from build123d import *

# Parameters (mm, degrees)
SKETCH_R              = 1.6
PAD_DEPTH             = 3
POLARPATTERN_COUNT    = 3
POCKET_DEPTH          = 380.288671
POLARPATTERN001_COUNT = 3
CHAMFER_SIZE          = 1
FILLET_R              = 3
SKETCH066_R           = 1.6
POCKET032_DEPTH       = 3.001
SKETCH078_R           = 3
POCKET038_DEPTH       = 5
POLARPATTERN007_COUNT = 3
CHAMFER017_SIZE       = 3


with BuildPart() as part:
    # Sketch → Pad (new body)
    with BuildSketch(Plane.XY):
        Polygon((0, 0), (-49.917704, 28.82), (-56.37248, 17.64), (-49.641016, 5.980762), (-58.30127, 0.980762), (-71.291651, -6.519238), (-41.291651, -58.480762), (-28.30127, -50.980762), (-19.641016, -45.980762), (-12.909552, -57.64), (0, -57.64), align=None)
        with Locations((-51.471143, -0.849365)):
            Circle(SKETCH_R, mode=Mode.SUBTRACT)
    pad = extrude(amount=PAD_DEPTH)

    # PolarPattern: Pad ×3 about axis
    polarpattern_axis = Axis((0, 0, 0), (0, 0, 1))
    for i in range(1, POLARPATTERN_COUNT):
        add(pad.rotate(polarpattern_axis, i * 360 / POLARPATTERN_COUNT))

    # Sketch001 → Pocket (cut, through all)
    with BuildSketch(Plane.XY):
        Polygon((-28.267069, 16.32), (-37.267069, 0.731543), (-18, -32.64), (0, -32.64), (0, 0), align=None)
    pocket = extrude(amount=POCKET_DEPTH, mode=Mode.SUBTRACT)

    # PolarPattern001: Pocket ×3 about axis
    polarpattern001_axis = Axis((0, 0, 0), (0, 0, 1))
    for i in range(1, POLARPATTERN001_COUNT):
        add(pocket.rotate(polarpattern001_axis, i * 360 / POLARPATTERN001_COUNT), mode=Mode.SUBTRACT)

    # Chamfer
    chamfer_edges = [part.edges().sort_by_distance(p)[0] for p in [
        (-56.37248, 17.64, 1.5),
        (-43.462928, 40, 1.5),
        (43.462928, 40, 1.5),
        (56.37248, 17.64, 1.5),
        (12.909552, -57.64, 1.5),
        (-12.909552, -57.64, 1.5),
    ]]
    chamfer(chamfer_edges, length=CHAMFER_SIZE)

    # Fillet
    fillet_edges = [part.edges().sort_by_distance(p)[0] for p in [
        (-19.267069, 31.908457, 1.5),
        (18, -32.64, 1.5),
        (-18, -32.64, 1.5),
        (37.267069, 0.731543, 1.5),
        (19.267069, 31.908457, 1.5),
        (-37.267069, 0.731543, 1.5),
    ]]
    fillet(fillet_edges, radius=FILLET_R)

    # Sketch066 (on Binder) → Pocket032 (cut, through all)
    with BuildSketch(Plane(origin=(0, 0, 3), x_dir=(1, 0, 0), z_dir=(0, 0, -1))):
        with Locations((-24.348373, 30.5)):
            Circle(SKETCH066_R)
        with Locations((38.587961, 5.836309)):
            Circle(SKETCH066_R)
        with Locations((-14.239588, -36.336309)):
            Circle(SKETCH066_R)
    extrude(amount=POCKET032_DEPTH, mode=Mode.SUBTRACT)

    # Sketch078 (on Face44 of Pocket032) → Pocket038 (cut)
    with BuildSketch(Plane.XY.offset(3)):
        with Locations((25, 45)):
            Circle(SKETCH078_R)
    pocket038 = extrude(amount=-POCKET038_DEPTH, mode=Mode.SUBTRACT)

    # PolarPattern007: Pocket038 ×3 about axis
    polarpattern007_axis = Axis((0, 0, 3), (0, 0, 1))
    for i in range(1, POLARPATTERN007_COUNT):
        add(pocket038.rotate(polarpattern007_axis, i * 360 / POLARPATTERN007_COUNT), mode=Mode.SUBTRACT)

    # Chamfer017
    chamfer017_edges = [part.edges().sort_by_distance(p)[0] for p in [
        (-41.291651, -58.480762, 1.5),
        (-71.291651, -6.519238, 1.5),
        (-30, 65, 1.5),
        (41.291651, -58.480762, 1.5),
        (71.291651, -6.519238, 1.5),
        (30, 65, 1.5),
        (-19.641016, -45.980762, 1.5),
        (49.641016, 5.980762, 1.5),
        (-30, 40, 1.5),
        (30, 40, 1.5),
        (-49.641016, 5.980762, 1.5),
        (19.641016, -45.980762, 1.5),
    ]]
    chamfer(chamfer017_edges, length=CHAMFER017_SIZE)


solid = part.part
Here's how the part is built. I have some questions about the finished solid (model axes, mm). A direction names the side the tool comes from. Round coordinates to 2 decimals unless told otherwise and drop trailing zeros. Write each loop counter-clockwise with the first axis right and the second up, starting at its lowest first coordinate (ties: lowest second). Pieces come first, ordered by that corner, then holes. Notation, with made-up numbers: (62.5, -5.5) -> (73.5, -5.5) arc R19 cw to (73.5, 26.5) -> close; hole circle Ø10 at (68.5, 60.5). An arc over 180 degrees is marked (long way). One line per item, written item: value.
1) We'd pull the mould along Y, two halves only. Please class faces 1 (the face through (28, 64, 1)), 2 (the face through (15.742, -52.734, 1.479)), 3 (the face through (-30, 53, 1)), 4 (the face through (-27.756, -15.742, 1.479)): released by +Y, released by -Y, zero draft, split by the parting line, or undercut.
Filled sheet:
face 1: released by +Y
face 2: released by -Y
face 3: zero draft
face 4: undercut
2) I'm going to push flat-ended pins straight in: pin 1 Ø0.5 at (y, z) = (18, 1.5) entering from +X; pin 2 Ø1.5 at (x, z) = (-39.5, 1.5) entering from +Y; pin 3 Ø1.5 at (y, z) = (-18.5, 1) entering from -X. Where does each tip first touch, or does it pass through?
Filled sheet:
pin 1: stops at x = 55.87
pin 2: stops at y = 40
pin 3: stops at x = -64.81
3) For faces 5 (the face through (38, 40, 1)), 6 (the face through (-38, 40, 1)), 7 (the face through (-53.54, 12.734, 1.479)), which set-ups out of +Z, -Z, +X, -X, +Y, -Y let a thin tool reach every point of the face, with its end or its side?
Filled sheet:
face 5: +Z, -Z, +X, +Y
face 6: +Z, -Z, -X, +Y
face 7: +Z, -Z, -X
4) Suppose I cut it at B-B on y = 45. List the corners of the cut face in (x, z) for me, plus the area to 3 significant figures.
Filled sheet:
outline: (-30, 0) -> (22, 0) -> (22, 3) -> (-30, 3) -> close; (28, 0) -> (30, 0) -> (30, 3) -> (28, 3) -> close
area: 162 mm2
5) If I drill on line 1 (Y direction, x = 25, z = 1.15); line 2 (Y direction, x = 17, z = 1.05); line 3 (Y direction, x = -55.5, z = 2.25), over which ranges is the centre line in solid material (lowest first)? Write a range as [from, to].
Filled sheet:
line 1: y = [-49.07, -46.77], [-41.54, -20.52], [21.98, 42], [48, 65]
line 2: y = [-50.56, -32.55], [31.91, 65]
line 3: y = [-33.87, 2.6], [16.13, 19.15]
6) Suppose I cut it at A-A on x = -8. List the corners of the cut face in (y, z) for me.
Filled sheet:
outline: (-57.64, 0) -> (-32.64, 0) -> (-32.64, 3) -> (-57.64, 3) -> close; (31.91, 0) -> (65, 0) -> (65, 3) -> (31.91, 3) -> close
